from build123d import *

# Parameters (mm, degrees)
BOSS_EXTRUDE1_DEPTH     = 415.925
F_1_4_CLEARANCE_HOLE1_D = 6.7564
LPATTERN1_COUNT         = 5
LPATTERN1_PITCH         = 171.45
F_10_CLEARANCE_HOLE2_D  = 5.1054


with BuildPart() as part:
    # Sketch1 → Boss-Extrude1 (new, symmetric)
    with BuildSketch(Plane(origin=(0, 0, 0), x_dir=(0, 0, -1), z_dir=(1, 0, 0))):
        with BuildLine():
            Line((0, 0), (50.8, 0))
            Line((50.8, 0), (50.8, -2.2225))
            ThreePointArc((50.8, -2.2225), (50.056051224, -4.018551224), (48.26, -4.7625))
            Line((48.26, -4.7625), (4.7625, -4.7625))
            Line((4.7625, -4.7625), (4.7625, -48.26))
            ThreePointArc((4.7625, -48.26), (4.018551224, -50.056051224), (2.2225, -50.8))
            Line((2.2225, -50.8), (0, -50.8))
            Line((0, -50.8), (0, 0))
        make_face()
    extrude(amount=BOSS_EXTRUDE1_DEPTH, both=True)

    # 1/4 Clearance Hole1 (through all)
    with Locations(Plane(origin=(0, 0, -4.7625), x_dir=(-1, 0, 0), z_dir=(0, 0, -1))):
        with Locations((-381, -17.4625), (-304.8, -38.1)):
            f_1_4_clearance_hole1 = Hole(F_1_4_CLEARANCE_HOLE1_D / 2)

    # LPattern1: 1/4 Clearance Hole1 ×5, 1 skipped
    with Locations(*[(-i * LPATTERN1_PITCH, 0, 0) for i in range(1, LPATTERN1_COUNT) if i not in (2,)]):
        add(f_1_4_clearance_hole1, mode=Mode.SUBTRACT)

    # #10 Clearance Hole2 (through all)
    with Locations(Plane(origin=(0, 0, 0), x_dir=(1, 0, 0), z_dir=(0, 1, 0))):
        with Locations((-34.925, 25.4), (-34.925, 38.1), (-212.725, 38.1), (-212.725, 25.4), (-390.525, 25.4), (-390.525, 38.1), (390.525, 38.1), (390.525, 25.4)):
            Hole(F_10_CLEARANCE_HOLE2_D / 2)


solid = part.part
For this review, take the finished solid that the model builds, in its own axes (mm). A direction names the side the tool comes from. Give positions to 0.01 mm unless a question says otherwise; leave off trailing zeros. Order: outer loops, then holes, each group sorted by start corner. A loop starts at its lowest first (then second) coordinate and runs counter-clockwise, first axis right, second up. Notation, with made-up numbers: M -34,58 L 7,58 A13 cw 7,83 Z; hole C 80,-21.5 d7. An arc over 180 degrees is marked long. Answer in a Markdown table with one row per item. Add a question column.
(1) Wall thickness on probe 1 along X at (y, z) = (-2, -38) (3 decimals); probe 2 along Z at (x, y) = (-341, -42): over which ranges is each line inside the solid? List them lowest first. Write a range as [from, to].
(2) Consider section B-B on z = -14. State the section outline as (x, y) points (1 decimal), and give its area (3 significant figures).
(3) Consider section A-A on x = 95. State the section outline as (y, z) points.
(4) For faces 1 (the face through (6, -26, 0)), 2 (the face through (6, -26, -4.762)), list the 3-axis set-ups (+Z, -Z, +X, -X, +Y, -Y) from which the entire face can be reached by the end or side of a thin tool; tool diameter is ignored.
(5) For pin 1 (2 mm diameter, centred on x = -233.5, z = -14.5, fed in from -Y); pin 2 (5.5 mm diameter, centred on x = 304.8, y = -38.1, fed in from -Z); pin 3 (12 mm diameter, centred on x = -133, y = -43.5, fed in from -Z), all flat-tipped, find the tip position at first contact; note any pin that passes through.
Evaluation:
| question | item | result |
|---|---|---|
| 1 | probe 1 | x = [-415.925, -393.076], [-387.974, -215.276], [-210.174, -37.476], [-32.374, 387.974], [393.076, 415.925] |
| 1 | probe 2 | z = [-4.76, 0] |
| 2 | outline | M -415.9,-4.8 L 415.9,-4.8 L 415.9,0 L -415.9,0 Z |
| 2 | area | 3,960 mm^2 |
| 3 | outline | M -50.8,-2.22 A2.54 ccw -48.26,-4.76 L -4.76,-4.76 L -4.76,-48.26 A2.54 ccw -2.22,-50.8 L 0,-50.8 L 0,0 L -50.8,0 Z |
| 4 | face 1 | +Z, +X, -X, +Y, -Y |
| 4 | face 2 | -Z, +X, -X, -Y |
| 5 | pin 1 | stops at y = -4.76 |
| 5 | pin 2 | passes through |
| 5 | pin 3 | stops at z = -4.76 |
